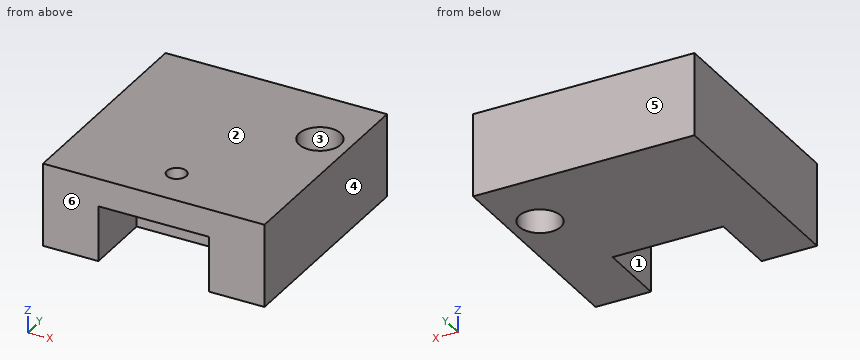
from build123d import *

# Parameters (mm, degrees)
SKETCH1_W           = 80
SKETCH1_H           = 80
BOSS_EXTRUDE1_DEPTH = 30
SKETCH3_W           = 40
SKETCH3_H           = 25
CUT_EXTRUDE2_DEPTH  = 20
SKETCH4_R           = 3.5
CUT_EXTRUDE3_DEPTH  = 61
SKETCH6_R           = 7.5
CUT_EXTRUDE5_DEPTH  = 65.031242374


with BuildPart() as part:
    # Sketch1 → Boss-Extrude1 (new body)
    with BuildSketch(Plane.XY):
        Rectangle(SKETCH1_W, SKETCH1_H)
    extrude(amount=BOSS_EXTRUDE1_DEPTH)

    # Sketch3 → Cut-Extrude2 (cut)
    with BuildSketch(Plane(origin=(0, 0, 0), x_dir=(-1, 0, 0), z_dir=(0, 0, -1))):
        with Locations((0, -27.5)):
            Rectangle(SKETCH3_W, SKETCH3_H)
    extrude(amount=-CUT_EXTRUDE2_DEPTH, mode=Mode.SUBTRACT)

    # Sketch4 → Cut-Extrude3 (cut, through all)
    with BuildSketch(Plane(origin=(0, 0, 20), x_dir=(-1, 0, 0), z_dir=(0, 0, -1))):
        with Locations((0, -25)):
            Circle(SKETCH4_R)
    extrude(amount=-CUT_EXTRUDE3_DEPTH, mode=Mode.SUBTRACT)

    # Sketch6 → Cut-Extrude5 (cut, through all)
    with BuildSketch(Plane.XY.offset(30)):
        with Locations((29.056312598, 16)):
            Circle(SKETCH6_R)
    extrude(amount=-CUT_EXTRUDE5_DEPTH, mode=Mode.SUBTRACT)


solid = part.part
Geometry: final body of the model. Coordinates: model frame, mm. Face numbers are marked on the shaded views. A direction names the side the tool comes from. Give positions to 0.01 mm unless a question says otherwise; leave off trailing zeros. Order: outer loops, then holes, each group sorted by start corner. A loop starts at its lowest first (then second) coordinate and runs counter-clockwise, first axis right, second up. Notation, with made-up numbers: (59, -37) -> (102, -37) arc R25 ccw to (102, -10) -> close; hole circle Ø8 at (28, 53.25). An arc over 180 degrees is marked (long way). Put each result on its own line as item: value.
Q1. Draft query along Y for the marked faces 3, 4, 5 and 6. Return one class per face: released by +Y, released by -Y, zero draft, split by the parting line, or undercut.
Here are the results:
face 3: undercut
face 4: zero draft
face 5: released by +Y
face 6: released by -Y
Q2. Material intervals for L1, parallel to Y at x = 29.5, z = 4.75; L2, parallel to Y at x = 0, z = 22.25; L3, parallel to X at y = -20, z = 16.5, sorted ascending.
Here are the results:
L1: y = -40 to 8.51, 23.49 to 40
L2: y = -40 to -28.5, -21.5 to 40
L3: x = -40 to -20, 20 to 40
Q3. Section A-A, the plane x = 0. Return loops of the section in (y, z), then the cut area to 3 significant figures.
Here are the results:
outline: (-40, 20) -> (-28.5, 20) -> (-28.5, 30) -> (-40, 30) -> close; (-21.5, 20) -> (-15, 20) -> (-15, 0) -> (40, 0) -> (40, 30) -> (-21.5, 30) -> close
area: 1,830 mm^2
Q4. Reachability of the marked faces 1 and 2 from +Z, -Z, +X, -X, +Y, -Y: full face, straight path, thin tool, end or side. Return the list, or none.
Here are the results:
face 1: -Z, -Y
face 2: +Z, +X, -X, +Y, -Y
Q5. Section D-D, the plane y = -32.5. Return loops of the section in (x, z).
Here are the results:
outline: (-40, 0) -> (-20, 0) -> (-20, 20) -> (20, 20) -> (20, 0) -> (40, 0) -> (40, 30) -> (-40, 30) -> close
Q6. Section C-C, the plane z = 14. Return loops of the section in (x, y), then the cut area to 3 significant figures.
Here are the results:
outline: (-40, -40) -> (-20, -40) -> (-20, -15) -> (20, -15) -> (20, -40) -> (40, -40) -> (40, 40) -> (-40, 40) -> close; hole circle Ø15 at (29.06, 16)
area: 5,220 mm^2
Q7. Pin query (flat end, axial travel): pin 1 (3 mm diameter, centred on x = 30.5, y = -14, fed in from -Z); pin 2 (6 mm diameter, centred on x = 1.5, z = 6, fed in from -Y). Return the tip coordinate at first contact, or that it passes through.
Here are the results:
pin 1: stops at z = 0
pin 2: stops at y = -15
Q8. Section B-B, the plane y = 16. Return loops of the section in (x, z), then the cut area to 3 significant figures.
Here are the results:
outline: (-40, 0) -> (21.56, 0) -> (21.56, 30) -> (-40, 30) -> close; (36.56, 0) -> (40, 0) -> (40, 30) -> (36.56, 30) -> close
area: 1,950 mm^2
